Input: part model. Units: mm. Frame: model coordinates. Round coordinates to 2 decimals unless told otherwise and drop trailing zeros. Loops run counter-clockwise (first coordinate to the right, second up) from the corner with the lowest first, then second, coordinate; pieces in that order, holes last.
(1) Cut plane A-A, the plane x = 0. Output: boundary loops of the cut face in (y, z), and give its area (3 significant figures).
(2) First-contact query: pin 1 Ø5 at (x, y) = (104.5, 20) entering from -Z; pin 2 Ø0.8 at (x, z) = (8.5, -0.5) entering from -Y; pin 3 Ø2 at (y, z) = (40.5, 1) entering from +X. Flat tips, straight axial feed; report the tip coordinate or a pass-through.
(3) Cut plane B-B, the plane y = 35. Output: boundary loops of the cut face in (x, z).
(4) Draft query along X for faces 1 (the face through (10, 3.2, 1.5)), 2 (the face through (123.252, 44.185, 1.479)), 3 (the face through (8, 69, 0)). Return one class per face: released by +X, released by -X, zero draft, split by the parting line, or undercut.
(5) Cut plane C-C, the plane z = 1.2. Give the number of separate pieces and of enclosed holes in the cut face, and give its area (3 significant figures).
(6) Line query: line 1 (Y direction, x = -24, z = 1.75); line 2 (Y direction, x = 108, z = 1.4); line 3 (X direction, y = 9, z = 1.9). Output: solid intervals per line, ascending.
(7) Cut plane D-D, the plane y = 113. Output: boundary loops of the cut face in (x, z), and give its area (3 significant figures).
from build123d import *
from build123d.topology import SkipClean

# Parameters (mm, degrees)
SKETCH1_R           = 10.5
SKETCH1_R_2         = 1.5
SKETCH1_W           = 8
SKETCH1_H           = 40
SKETCH1_R_3         = 5
BOSS_EXTRUDE1_DEPTH = 3
CUT_EXTRUDE1_REACH  = 140.687
SKETCH2_R           = 2
BOSS_EXTRUDE2_DEPTH = 3
SKETCH4_W           = 2
SKETCH4_H           = 6.5
SKETCH4_W_2         = 6.5
SKETCH4_H_2         = 2
BOSS_EXTRUDE3_DEPTH = 1
SKETCH5_R           = 2
CUT_EXTRUDE2_DEPTH  = 10
BOSS_EXTRUDE4_START = -3
BOSS_EXTRUDE4_DEPTH = 3
SKETCH7_R           = 2
CUT_EXTRUDE3_DEPTH  = 10
BOSS_EXTRUDE5_START = -3
SKETCH8_R           = 65
SKETCH8_R_2         = 10.5
BOSS_EXTRUDE5_DEPTH = 3
CUT_EXTRUDE4_START  = -10
CUT_EXTRUDE4_DEPTH  = 10
CUT_EXTRUDE5_REACH  = 237.883
SKETCH10_R          = 1.5


with BuildPart() as part:
    # Sketch1 → Boss-Extrude1 (new body)
    # profile 1 of 2: a face of its own
    with BuildSketch(Plane.XY):
        with BuildLine():
            ThreePointArc((-60, 0), (-52.867640737, 28.372743309), (-33.166247904, 50))
            Line((-33.166247904, 50), (-60, 50))
            Line((-60, 50), (-60, 0))
        make_face()
    # profile 2 of 2: a face of its own
    with BuildSketch(Plane.XY):
        with BuildLine():
            ThreePointArc((0, 60), (-17.320508076, 57.445626465), (-33.166247904, 50))
            ThreePointArc((-33.166247904, 50), (-52.867640737, 28.372743309), (-60, 0))
            ThreePointArc((-60, 0), (-15.529142706, -57.955549577), (51.961524227, -30))
            Line((51.961524227, -30), (56.882127578, -30))
            Line((56.882127578, -30), (90, -30))
            Line((90, -30), (90, -10.355339059))
            Line((90, -10.355339059), (117.67766953, 17.32233047))
            ThreePointArc((117.67766953, 17.32233047), (123.096988313, 44.567085809), (100, 60))
            Line((100, 60), (0, 60))
        make_face()
        Circle(SKETCH1_R, mode=Mode.SUBTRACT)
        with Locations((69, -26)):
            Circle(SKETCH1_R_2, mode=Mode.SUBTRACT)
        with Locations((76, 0)):
            Rectangle(SKETCH1_W, SKETCH1_H, mode=Mode.SUBTRACT)
        with Locations((83, -26)):
            Circle(SKETCH1_R_2, mode=Mode.SUBTRACT)
        with Locations((100, 35)):
            Circle(SKETCH1_R_3, mode=Mode.SUBTRACT)
    extrude(amount=BOSS_EXTRUDE1_DEPTH)

    # Sketch2 → Cut-Extrude1 (cut, up to next)
    with BuildSketch(Plane.XY.offset(3), mode=Mode.PRIVATE) as cut_extrude1_sk1:
        with Locations((60, 45)):
            Circle(SKETCH2_R)
    cut_extrude1_tool1 = extrude(cut_extrude1_sk1.sketch, amount=-CUT_EXTRUDE1_REACH, mode=Mode.PRIVATE) & part.part
    add(cut_extrude1_tool1.solids().sort_by_distance((60, 45, 3))[0], mode=Mode.SUBTRACT)

    # Sketch3 → Boss-Extrude2 (add)
    with BuildSketch(Plane(origin=(0, 0, 0), x_dir=(-1, 0, 0), z_dir=(0, 0, -1))):
        with BuildLine():
            Line((-30, 80), (-30, 60))
            Line((-30, 60), (0, 60))
            ThreePointArc((0, 60), (2.502176759, 59.947803225), (5, 59.791303716))
            Line((5, 59.791303716), (5, 80))
            Line((5, 80), (-30, 80))
        make_face()
    extrude(amount=-BOSS_EXTRUDE2_DEPTH)

    # Sketch4 → Boss-Extrude3 (add)
    with BuildSketch(Plane(origin=(0, 0, 0), x_dir=(-1, 0, 0), z_dir=(0, 0, -1))):
        with Locations((-12.5, 68.846087829)):
            Rectangle(SKETCH4_W, SKETCH4_H)
        with Locations((-16.75, 64.596087829)):
            Rectangle(SKETCH4_W_2, SKETCH4_H_2)
        with Locations((-12.5, 64.596087829)):
            Rectangle(SKETCH4_W, SKETCH4_H_2)
        with Locations((-8.25, 64.596087829)):
            Rectangle(SKETCH4_W_2, SKETCH4_H_2)
        with Locations((-12.5, 60.346087829)):
            Rectangle(SKETCH4_W, SKETCH4_H)
    extrude(amount=BOSS_EXTRUDE3_DEPTH)

    # Sketch5 → Cut-Extrude2 (cut)
    with BuildSketch(Plane.XY.offset(3)):
        with Locations((92, 43)):
            Circle(SKETCH5_R)
        with Locations((108, 43)):
            Circle(SKETCH5_R)
        with Locations((108, 27)):
            Circle(SKETCH5_R)
        with Locations((92, 27)):
            Circle(SKETCH5_R)
    extrude(amount=-CUT_EXTRUDE2_DEPTH, mode=Mode.SUBTRACT)

    # Sketch6 → Boss-Extrude4 (add)
    with BuildSketch(Plane.XY.offset(3).offset(BOSS_EXTRUDE4_START)):
        with BuildLine():
            Line((12.5, 60), (55, 60))
            Line((55, 60), (55, 200))
            Line((55, 200), (-30, 200))
            Line((-30, 200), (-30, 60))
            Line((-30, 60), (-30, 51.961524227))
            ThreePointArc((-30, 51.961524227), (-17.93255034, 57.257520364), (-5, 59.791303716))
            Line((-5, 59.791303716), (-5, 60))
            Line((-5, 60), (12.5, 60))
        make_face()
    extrude(amount=BOSS_EXTRUDE4_DEPTH)

    # Sketch7 → Cut-Extrude3 (cut)
    with BuildSketch(Plane.XY.offset(3)):
        with Locations((-24, 194.5)):
            Circle(SKETCH7_R)
        with Locations((49, 194.5)):
            Circle(SKETCH7_R)
        with Locations((49, 65.5)):
            Circle(SKETCH7_R)
        with Locations((-24, 65.5)):
            Circle(SKETCH7_R)
        with Locations((-24, 130)):
            Circle(SKETCH7_R)
        with Locations((49, 130)):
            Circle(SKETCH7_R)
    extrude(amount=-CUT_EXTRUDE3_DEPTH, mode=Mode.SUBTRACT)

    # Sketch8 → Boss-Extrude5 (add)
    with BuildSketch(Plane.XY.offset(3).offset(BOSS_EXTRUDE5_START)):
        Circle(SKETCH8_R)
        Circle(SKETCH8_R_2, mode=Mode.SUBTRACT)
    extrude(amount=BOSS_EXTRUDE5_DEPTH)

    # Sketch9 → Cut-Extrude4 (cut)
    with SkipClean():  # the faces are left unmerged after this step: merging them gives an invalid solid
        with BuildSketch(Plane.XY.offset(3).offset(CUT_EXTRUDE4_START)):
            with BuildLine():
                Line((-60, 50), (-60, 25))
                ThreePointArc((-60, 25), (-52.282822987, 38.62002616), (-41.533119315, 50))
                Line((-41.533119315, 50), (-60, 50))
            make_face()
        extrude(amount=CUT_EXTRUDE4_DEPTH, mode=Mode.SUBTRACT)

    # Sketch10 → Cut-Extrude5 (cut, up to next)
    with BuildSketch(Plane.XY.offset(3), mode=Mode.PRIVATE) as cut_extrude5_sk1:
        with Locations((-15, 25.980762114)):
            Circle(SKETCH10_R)
    cut_extrude5_tool1 = extrude(cut_extrude5_sk1.sketch, amount=-CUT_EXTRUDE5_REACH, mode=Mode.PRIVATE) & part.part
    # Sketch10 → Cut-Extrude5 (cut, up to next)
    with BuildSketch(Plane.XY.offset(3), mode=Mode.PRIVATE) as cut_extrude5_sk2:
        with Locations((-25.980762114, -15)):
            Circle(SKETCH10_R)
    cut_extrude5_tool2 = extrude(cut_extrude5_sk2.sketch, amount=-CUT_EXTRUDE5_REACH, mode=Mode.PRIVATE) & part.part
    # Sketch10 → Cut-Extrude5 (cut, up to next)
    with BuildSketch(Plane.XY.offset(3), mode=Mode.PRIVATE) as cut_extrude5_sk3:
        with Locations((15, -25.980762114)):
            Circle(SKETCH10_R)
    cut_extrude5_tool3 = extrude(cut_extrude5_sk3.sketch, amount=-CUT_EXTRUDE5_REACH, mode=Mode.PRIVATE) & part.part
    # Sketch10 → Cut-Extrude5 (cut, up to next)
    with BuildSketch(Plane.XY.offset(3), mode=Mode.PRIVATE) as cut_extrude5_sk4:
        with Locations((96.767766953, 10.554563517)):
            Circle(SKETCH10_R)
    cut_extrude5_tool4 = extrude(cut_extrude5_sk4.sketch, amount=-CUT_EXTRUDE5_REACH, mode=Mode.PRIVATE) & part.part
    add(cut_extrude5_tool1.solids().sort_by_distance((-15, 25.980762, 3))[0], mode=Mode.SUBTRACT)
    add(cut_extrude5_tool2.solids().sort_by_distance((-25.980762, -15, 3))[0], mode=Mode.SUBTRACT)
    add(cut_extrude5_tool3.solids().sort_by_distance((15, -25.980762, 3))[0], mode=Mode.SUBTRACT)
    add(cut_extrude5_tool4.solids().sort_by_distance((96.767767, 10.554564, 3))[0], mode=Mode.SUBTRACT)


solid = part.part
Reported:
1. outline: (-65, 0) - (-10.5, 0) - (-10.5, 3) - (-65, 3) - close; (10.5, 0) - (200, 0) - (200, 3) - (10.5, 3) - close
1. area: 732 mm2
2. pin 1: stops at z = 0
2. pin 2: stops at y = 63.6
2. pin 3: stops at x = 124.59
3. outline: (-54.77, 0) - (95, 0) - (95, 3) - (-54.77, 3) - close; (105, 0) - (125, 0) - (125, 3) - (105, 3) - close
4. face 1: undercut
4. face 2: released by +X
4. face 3: zero draft
5. separate pieces: 1
5. enclosed holes: 20
5. area: 28,800 mm2
6. line 1: y = -60.41 to 63.5, 67.5 to 128, 132 to 192.5, 196.5 to 200
6. line 2: y = 7.64 to 25, 29 to 41, 45 to 58.69
6. line 3: x = -64.37 to -5.41, 5.41 to 72, 80 to 109.36
7. outline: (-30, 0) - (55, 0) - (55, 3) - (-30, 3) - close
7. area: 255 mm2
